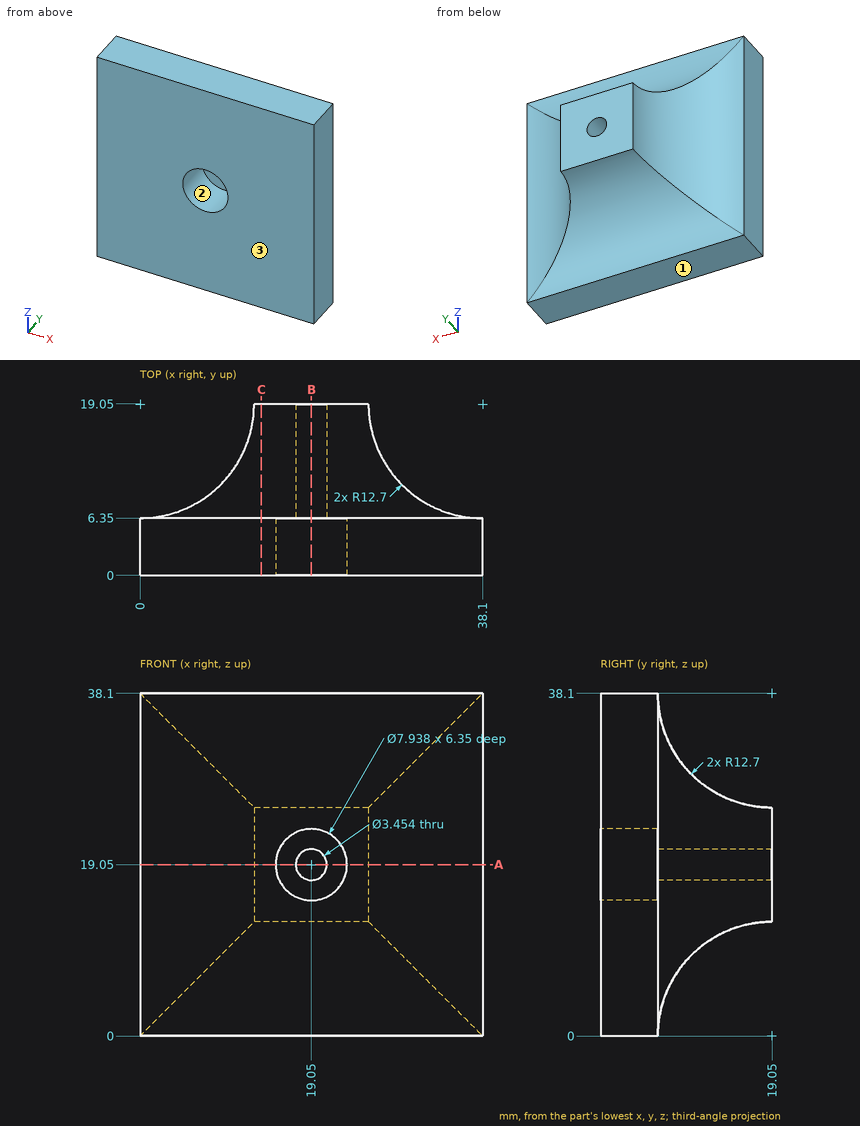
Drawing for the job (mm, zero at the part's lowest x, y, z). Round coordinates to 2 decimals unless told otherwise and drop trailing zeros. Order: outer loops, then holes, each group sorted by start corner. A loop starts at its lowest first (then second) coordinate and runs counter-clockwise, first axis right, second up. Notation, with made-up numbers: (54.25, -7.75) -> (63.25, -7.75) arc R25 ccw to (63.25, 27.25) -> close; hole circle Ø5 at (57.25, -5.75). An arc over 180 degrees is marked (long way). Write item = value, one per line. Start each with the question number.
(1) Cut at B-B, the plane x = 19.05. List the corners of the cut face in (y, z), then the cut area to 3 significant figures.
(2) Pin check, flat tips, straight feed: P1, Ø1, axis at x = 21.5, y = 11, coming from the -Z side; P2, Ø3, axis at x = 15, y = 17, coming from the +Z side; P3, Ø2.5, axis at x = 21, z = 19, coming from the -Y side. Stop position of each tip, or through.
(3) Probe line 1 (Z direction, x = 19.05, y = 2.75); line 2 (Y direction, x = 17.5, z = 15.5); line 3 (Z direction, x = 20.5, y = 12.75) (1 decimal). List the from-to ranges inside material, lowest first. Write a range as [from, to].
(4) Pull direction Z, two halves, no side cores. Call the marked faces 1, 2 and 3: released by +Z, released by -Z, zero draft, split by the parting line, or undercut.
(5) Cut at A-A, the plane z = 19.05. List the corners of the cut face in (x, y).
(6) Cut at C-C, the plane x = 13.5. List the corners of the cut face in (y, z).
Model answer:
q1.outline = (0, 0) -> (6.35, 0) arc R12.7 cw to (19.05, 12.7) -> (19.05, 17.32) -> (6.35, 17.32) -> (6.35, 15.08) -> (0, 15.08) -> close; (0, 23.02) -> (6.35, 23.02) -> (6.35, 20.78) -> (19.05, 20.78) -> (19.05, 25.4) arc R12.7 cw to (6.35, 38.1) -> (0, 38.1) -> close
q1.area = 378 mm2
q2.P1 = 9.39
q2.P2 = 25.91
q2.P3 = 6.35
q3.line_1 = [0, 15.08], [23.02, 38.1]
q3.line_2 = [6.35, 19.05]
q3.line_3 = [11, 18.1], [20, 27.1]
q4.face_1 = released by -Z
q4.face_2 = undercut
q4.face_3 = zero draft
q5.outline = (0, 0) -> (15.08, 0) -> (15.08, 6.35) -> (17.32, 6.35) -> (17.32, 19.05) -> (12.7, 19.05) arc R12.7 cw to (0, 6.35) -> close; (20.78, 6.35) -> (23.02, 6.35) -> (23.02, 0) -> (38.1, 0) -> (38.1, 6.35) arc R12.7 cw to (25.4, 19.05) -> (20.78, 19.05) -> close
q6.outline = (0, 0) -> (6.35, 0) arc R12.7 cw to (19.05, 12.7) -> (19.05, 25.4) arc R12.7 cw to (6.35, 38.1) -> (0, 38.1) -> close
